Geometry check sheet. Reference: the model listing, model coordinates, mm. Face numbers are marked on the shaded views. A direction names the side the tool comes from. Give positions to 0.01 mm unless a question says otherwise; leave off trailing zeros. Loops run counter-clockwise (first coordinate to the right, second up) from the corner with the lowest first, then second, coordinate; pieces in that order, holes last.
1. Go/stop test with flat-tipped pins: pin 1 Ø5 at (x, y) = (51, 65.25) entering from -Z; pin 2 Ø2.5 at (y, z) = (58.25, 78.5) entering from +X; pin 3 Ø1.5 at (x, y) = (70, 67) entering from -Z. Record where each tip stops, or that it passes through.
2. Release check for a two-part mould opening along X. For the marked faces 4, 5 and 6 record: +X half, -X half, draft (parallel to the pull), parting line (faces both ways), or undercut.
3. Cross-section at D-D, the plane x = -64.5. Record the cut outline in (y, z), plus the area to 3 significant figures.
4. Material ranges on L1, parallel to Z at x = 75.8, y = 58.25; L2, parallel to X at y = -25, z = 22.5; L3, parallel to X at y = -64, z = 96, recorded low to high.
5. Cross-section at B-B, the plane y = 49. Record the cut outline in (x, z).
6. Cross-section at C-C, the plane y = -64.5. Record the cut outline in (x, z).
7. Cross-section at A-A, the plane z = 22. Record the cut outline in (x, y).
8. Tool access check on the marked faces 1, 2 and 3. Record the directions out of +Z, -Z, +X, -X, +Y, -Y that give a thin tool (end or side, any length) a straight path to the whole face; none if there is none.
from build123d import *

# Parameters (mm, degrees)
F1_DEPTH = 69
F2_R     = 2
F3_DEPTH = 3
F4_R     = 2
F5_DEPTH = 3
F7_DEPTH = 3


with BuildPart() as f1:
    # F0 (on Front) → F1 (new body, symmetric)
    with BuildSketch(Plane.XZ):
        Polygon((-76.5, 0), (-73.5, 0), (-73.5, 94), (0, 94), (73.5, 94), (73.5, 0), (76.5, 0), (76.5, 97), (0, 97), (-76.5, 97), align=None)
    extrude(amount=F1_DEPTH, both=True)

    # F2 (on face) → F3 (cut, through all)
    with BuildSketch(Plane.YZ.offset(76.5)):
        Polygon((53.5, 87), (28.5, 87), (3.5, 87), (3.5, 70), (28.5, 70), (53.5, 70), align=None)
        with Locations((-1.25, 78.5)):
            Circle(F2_R)
        with Locations((58.25, 78.5)):
            Circle(F2_R)
        with Locations((-1.25, 43.5)):
            Circle(F2_R)
        Polygon((28.5, 52), (3.5, 52), (3.5, 35), (28.5, 35), (53.5, 35), (53.5, 52), align=None)
        with Locations((58.25, 43.5)):
            Circle(F2_R)
    extrude(amount=-F3_DEPTH, mode=Mode.SUBTRACT)

    # F4 (on face) → F5 (cut, through all)
    with BuildSketch(Plane.XY.offset(97)):
        with Locations((-53.5, 65.25)):
            Circle(F4_R)
        with Locations((17.3, 65.25)):
            Circle(F4_R)
        with Locations((51, 65.25)):
            Circle(F4_R)
        with Locations((-64.5, -64.5)):
            Circle(F4_R)
        with Locations((20, -64.5)):
            Circle(F4_R)
        with Locations((67, -64.5)):
            Circle(F4_R)
        with Locations((34.5, -16)):
            Circle(F4_R)
        with Locations((52.5, -16)):
            Circle(F4_R)
        with Locations((52.5, -59)):
            Circle(F4_R)
        with Locations((34.5, -59)):
            Circle(F4_R)
    extrude(amount=-F5_DEPTH, mode=Mode.SUBTRACT)

    # F6 (on face) → F7 (join)
    with BuildSketch(Plane(origin=(0, 69, 0), x_dir=(-1, 0, 0), z_dir=(0, 1, 0))):
        with BuildLine():
            Line((-61.5, 97), (-76.5, 97))
            Line((-76.5, 97), (-76.5, 77))
            Line((-76.5, 77), (-68.5, 77))
            ThreePointArc((-68.5, 77), (-63.5502525317, 79.0502525317), (-61.5, 84))
            Line((-61.5, 84), (-61.5, 97))
        make_face()
    extrude(amount=-F7_DEPTH)


solid = f1.part
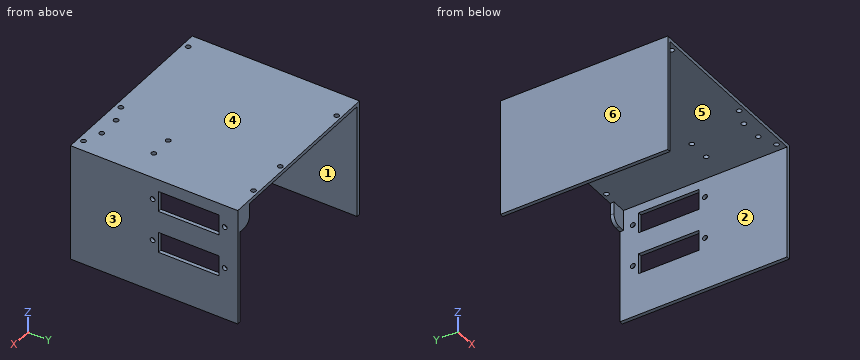
Result:
1. pin 1: stops at z = 94
1. pin 2: stops at x = -73.5
1. pin 3: stops at z = 77
2. face 4: draft
2. face 5: undercut
2. face 6: -X half
3. outline: (-69, 94) - (-66.5, 94) - (-66.5, 97) - (-69, 97) - close; (-62.5, 94) - (69, 94) - (69, 97) - (-62.5, 97) - close
3. area: 402 mm2
4. L1: z = 0 to 41.5, 45.5 to 76.5, 80.5 to 97
4. L2: x = -76.5 to -73.5, 73.5 to 76.5
4. L3: x = -76.5 to -66.44, -62.56 to 18.06, 21.94 to 65.06, 68.94 to 76.5
5. outline: (-76.5, 0) - (-73.5, 0) - (-73.5, 94) - (73.5, 94) - (73.5, 87) - (76.5, 87) - (76.5, 97) - (-76.5, 97) - close; (73.5, 0) - (76.5, 0) - (76.5, 35) - (73.5, 35) - close; (73.5, 52) - (76.5, 52) - (76.5, 70) - (73.5, 70) - close
6. outline: (-76.5, 0) - (-73.5, 0) - (-73.5, 94) - (-66.5, 94) - (-66.5, 97) - (-76.5, 97) - close; (-62.5, 94) - (18, 94) - (18, 97) - (-62.5, 97) - close; (22, 94) - (65, 94) - (65, 97) - (22, 97) - close; (69, 94) - (73.5, 94) - (73.5, 0) - (76.5, 0) - (76.5, 97) - (69, 97) - close
7. outline: (-76.5, -69) - (-73.5, -69) - (-73.5, 69) - (-76.5, 69) - close; (73.5, -69) - (76.5, -69) - (76.5, 69) - (73.5, 69) - close
8. face 1: -Z, +Y, -Y
8. face 2: -Z, -Y
8. face 3: +Z, -Z, +X, +Y, -Y
